Check sheet for the modelled part. Datum: model origin and axes. Units: mm. Coordinates: 2 decimals unless noted, no trailing zeros. Write each loop counter-clockwise with the first axis right and the second up, starting at its lowest first coordinate (ties: lowest second). Pieces come first, ordered by that corner, then holes. Notation, with made-up numbers: (86, 61) - (109, 61) arc R9 cw to (109, 74) - close; hole circle Ø9 at (-10, 88.5). An arc over 180 degrees is marked (long way). Write each question's results on one line, items separated by ' | '.
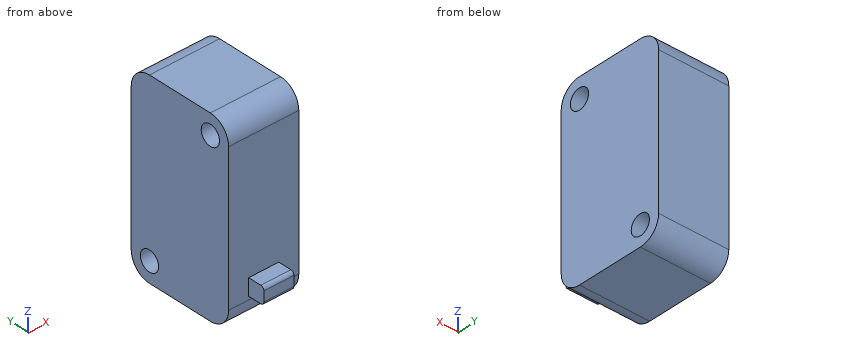
from build123d import *

# Parameters (mm, degrees)
SKETCH1_W           = 28
SKETCH1_H           = 16
BOSS_EXTRUDE1_DEPTH = 10.5
SKETCH2_R           = 1.5
CUT_EXTRUDE1_DEPTH  = 20.241881405
FILLET1_R           = 3
SKETCH3_W           = 4.5
SKETCH3_H           = 2.5
BOSS_EXTRUDE2_DEPTH = 2.5
FILLET2_R           = 0.5


with BuildPart() as part:
    # Sketch1 → Boss-Extrude1 (new body)
    with BuildSketch(Plane(origin=(0, 0, 0), x_dir=(0, 0, -1), z_dir=(1, 0, 0))):
        Rectangle(SKETCH1_W, SKETCH1_H)
    extrude(amount=BOSS_EXTRUDE1_DEPTH)

    # Sketch2 → Cut-Extrude1 (cut, through all)
    with BuildSketch(Plane(origin=(10.5, 0, 0), x_dir=(0, 0, -1), z_dir=(1, 0, 0))):
        with Locations((11, 5)):
            Circle(SKETCH2_R)
        with Locations((-11, -5)):
            Circle(SKETCH2_R)
    extrude(amount=-CUT_EXTRUDE1_DEPTH, mode=Mode.SUBTRACT)

    # Fillet1
    fillet1_edges = [part.edges().sort_by_distance(p)[0] for p in [
        (5.25, -8, -14),
        (5.25, -8, 14),
        (5.25, 8, 14),
        (5.25, 8, -14),
    ]]
    fillet(fillet1_edges, radius=FILLET1_R)

    # Sketch3 → Boss-Extrude2 (add)
    with BuildSketch(Plane.XZ.offset(8)):
        with Locations((5.25, -9.25)):
            Rectangle(SKETCH3_W, SKETCH3_H)
    extrude(amount=BOSS_EXTRUDE2_DEPTH)

    # Fillet2
    fillet2_edges = [part.edges().sort_by_distance(p)[0] for p in [
        (5.25, -10.5, -10.5),
        (5.25, -10.5, -8),
    ]]
    fillet(fillet2_edges, radius=FILLET2_R)


solid = part.part
1. Go/stop test with flat-tipped pins: pin 1 (0.8 mm diameter, centred on y = -9.5, z = -9.5, fed in from +X); pin 2 (0.6 mm diameter, centred on x = 6.5, y = -9, fed in from +Z); pin 3 (3 mm diameter, centred on x = 5.5, z = -2, fed in from -Y). Record where each tip stops, or that it passes through.
Values follow:
pin 1: stops at x = 7.5 | pin 2: stops at z = -8 | pin 3: stops at y = -8
2. Sectioned sample at B-B (x = 8.75). Record the cut outline in (y, z), then the cut area to 3 significant figures.
Values follow:
outline: (-8, -11) arc R3 ccw to (-5, -14) - (5, -14) arc R3 ccw to (8, -11) - (8, 11) arc R3 ccw to (5, 14) - (-5, 14) arc R3 ccw to (-8, 11) - close; hole circle Ø3 at (-5, 11); hole circle Ø3 at (5, -11) | area: 426 mm^2
3. Material ranges on L1, parallel to Y at x = 4.25, z = -11; L2, parallel to Y at x = 3, z = 11; L3, parallel to X at y = -9.5, z = -8.25, recorded low to high. Write a range as [from, to].
Values follow:
L1: y = [-8, 3.5], [6.5, 8] | L2: y = [-8, -6.5], [-3.5, 8] | L3: x = [3, 7.5]
4. Sectioned sample at A-A (z = -11.75). Record the cut outline in (x, y).
Values follow:
outline: (0, -7.9) - (10.5, -7.9) - (10.5, 3.7) - (0, 3.7) - close; (0, 6.3) - (10.5, 6.3) - (10.5, 7.9) - (0, 7.9) - close
5. Sectioned sample at C-C (z = 9). Record the cut outline in (x, y), then the cut area to 3 significant figures.
Values follow:
outline: (0, -8) - (10.5, -8) - (10.5, 8) - (0, 8) - close | area: 168 mm^2
